```python
from build123d import *

# Parameters (mm, degrees)
SKETCH1_R           = 25.4
BOSS_EXTRUDE1_DEPTH = 7.9375
SKETCH2_R           = 17.4625
BOSS_EXTRUDE2_DEPTH = 17.4625
CUT_EXTRUDE1_DEPTH  = 44.994090512
SKETCH4_R           = 2.413
CUT_EXTRUDE2_DEPTH  = 40.940692361
CIRPATTERN1_COUNT   = 6


with BuildPart() as part:
    # Sketch1 → Boss-Extrude1 (new body)
    with BuildSketch(Plane(origin=(0, 0, 0), x_dir=(1, 0, 0), z_dir=(0, 1, 0))):
        with Locations(Location((0, 0, 0), (0, 0, 270))):
            Circle(SKETCH1_R)
    extrude(amount=BOSS_EXTRUDE1_DEPTH)

    # Sketch2 → Boss-Extrude2 (add)
    with BuildSketch(Plane(origin=(0, 7.9375, 0), x_dir=(1, 0, 0), z_dir=(0, 1, 0))):
        with Locations(Location((0, 0, 0), (0, 0, 270))):
            Circle(SKETCH2_R)
    extrude(amount=BOSS_EXTRUDE2_DEPTH)

    # Sketch3 → Cut-Extrude1 (cut, through all)
    with BuildSketch(Plane(origin=(0, 25.4, 0), x_dir=(1, 0, 0), z_dir=(0, 1, 0))):
        with BuildLine():
            Line((-1.5875, 7.735861062), (1.5875, 7.735861062))
            Line((1.5875, 7.735861062), (1.5875, 6.148361062))
            ThreePointArc((1.5875, 6.148361062), (6.326022598, -0.551305799), (0.5, -6.330284354))
            Line((0.5, -6.330284354), (0.5, -25.4))
            Line((0.5, -25.4), (-0.5, -25.4))
            Line((-0.5, -25.4), (-0.5, -6.330284354))
            ThreePointArc((-0.5, -6.330284354), (-6.326022598, -0.551305799), (-1.5875, 6.148361062))
            Line((-1.5875, 6.148361062), (-1.5875, 7.735861062))
        make_face()
    extrude(amount=-CUT_EXTRUDE1_DEPTH, mode=Mode.SUBTRACT)

    # Sketch4 → Cut-Extrude2 (cut, through all)
    with BuildSketch(Plane(origin=(0, 7.9375, 0), x_dir=(1, 0, 0), z_dir=(0, 1, 0))):
        with Locations(Location((-21.43125, 0, 0), (0, 0, 270))):
            Circle(SKETCH4_R)
    cut_extrude2 = extrude(amount=-CUT_EXTRUDE2_DEPTH, mode=Mode.SUBTRACT)

    # CirPattern1: Cut-Extrude2 ×6 about axis
    cirpattern1_axis = Axis((0, 0, 0), (0, 1, 0))
    for i in range(1, CIRPATTERN1_COUNT):
        add(cut_extrude2.rotate(cirpattern1_axis, i * 360 / CIRPATTERN1_COUNT), mode=Mode.SUBTRACT)


solid = part.part
```
CAD build for the part. Positions are in the model's coordinates, mm. A direction names the side the tool comes from. Give positions to 0.01 mm unless a question says otherwise; leave off trailing zeros. Write each loop counter-clockwise with the first axis right and the second up, starting at its lowest first coordinate (ties: lowest second). Pieces come first, ordered by that corner, then holes. Notation, with made-up numbers: M 6.25,55.25 L 60.25,55.25 A26 ccw 60.25,84.25 Z; hole C 67.5,59 d6. An arc over 180 degrees is marked long. Return JSON: item names as keys, results as strings. Group by question number.
(1) Band-saw the part on A-A (z = 0). Give the cut face in (x, y), and give its area (3 significant figures).
(2) Flat gauge pins, fed straight in: pin 1 Ø6 at (x, z) = (17.5, 17.5) entering from +Y; pin 2 Ø2.5 at (x, y) = (-0.5, 16) entering from +Z; pin 3 Ø3 at (y, z) = (9.5, -2) entering from +X; pin 4 Ø3 at (x, z) = (-21.43, 0) entering from -Y. Where does each tip first touch, or does it go through?
(3) 3-axis set-ups, long thin cutter, end or side, ignore diameter. For faces 1 (the face through (-5, 0, -6)), 2 (the face through (1.588, 13, -7)), 3 (the face through (-17, 7.938, 6)), 4 (the face through (-0.5, 10, 14)): which of +Z, -Z, +X, -X, +Y, -Y reach the whole face in a straight line?
(4) Band-saw the part on D-D (x = -9.5). Give the cut face in (y, z), and give its area (3 significant figures).
(5) Mould opens along Z. For faces 5 (the face through (1.11, 3.913, -25.376)), 6 (the face through (-8, 25.4, 0)), 7 (the face through (-19.8, 4.02, -1.78)) say: pulls with the +Z half, pulls with the -Z half, needs draft (parallel to the pull), parting line crosses it, or undercut.
(6) Band-saw the part on C-C (x = 3). Give the cut face in (y, z), and give its area (3 significant figures).
(7) Drill centre lines: L1, parallel to X at y = 3.25, z = 0; L2, parallel to Y at x = -14, z = -11; L3, parallel to X at y = 17, z = 3.5. Where is each one in solid material? Low to high. Write a range as [from, to].
Entries:
{
 "1": {"outline": "M -25.4,0 L -23.84,0 L -23.84,7.94 L -25.4,7.94 Z; M -19.02,0 L -6.35,0 L -6.35,25.4 L -17.46,25.4 L -17.46,7.94 L -19.02,7.94 Z; M 6.35,0 L 19.02,0 L 19.02,7.94 L 17.46,7.94 L 17.46,25.4 L 6.35,25.4 Z; M 23.84,0 L 25.4,0 L 25.4,7.94 L 23.84,7.94 Z", "area": "614 mm^2"},
 "2": {"pin 1": "stops at y = 7.94", "pin 2": "stops at z = 17.46", "pin 3": "stops at x = 17.46", "pin 4": "passes through"},
 "3": {"face 1": "+Z, -Z, +X, -X, -Y", "face 2": "+Y, -Y", "face 3": "+Y", "face 4": "+Z, +Y, -Y"},
 "4": {"outline": "M 0,-23.56 L 7.94,-23.56 L 7.94,-20.64 L 0,-20.64 Z; M 0,-16.48 L 7.94,-16.48 L 7.94,-14.65 L 25.4,-14.65 L 25.4,14.65 L 7.94,14.65 L 7.94,16.48 L 0,16.48 Z; M 0,20.64 L 7.94,20.64 L 7.94,23.56 L 0,23.56 Z", "area": "820 mm^2"},
 "5": {"face 5": "parting line crosses it", "face 6": "needs draft", "face 7": "undercut"},
 "6": {"outline": "M 0,-25.22 L 7.94,-25.22 L 7.94,-17.2 L 25.4,-17.2 L 25.4,-5.6 L 0,-5.6 Z; M 0,5.6 L 25.4,5.6 L 25.4,17.2 L 7.94,17.2 L 7.94,25.22 L 0,25.22 Z", "area": "717 mm^2"},
 "7": {"L1": "x = [-25.4, -23.84], [-19.02, -6.35], [6.35, 19.02], [23.84, 25.4]", "L2": "y = [0, 7.94]", "L3": "x = [-17.11, -5.3], [5.3, 17.11]"}
}
